Read the model definition and answer for the solid it produces. Units are mm, in the model's axes. A direction names the side the tool comes from. Give positions to 0.01 mm unless a question says otherwise; leave off trailing zeros. Order: outer loops, then holes, each group sorted by start corner. A loop starts at its lowest first (then second) coordinate and runs counter-clockwise, first axis right, second up. Notation, with made-up numbers: (62, 20) - (101, 20) arc R3 ccw to (101, 25) - close; hole circle Ø6 at (68.25, 35.5). An arc over 180 degrees is marked (long way). Answer as CSV lines item,"result". Start each with the question number.
from build123d import *

# Parameters (mm, degrees)
BOSS_EXTRUDE2_DEPTH = 5


with BuildPart() as part:
    # Sketch1 → Boss-Extrude2 (new body)
    with BuildSketch(Plane.XY):
        with BuildLine():
            Line((-28.5, 0), (-25.5, 0))
            ThreePointArc((-25.5, 0), (-24.417654986, 7.350382643), (-21.2625, 14.076792737))
            Line((-21.2625, 14.076792737), (-21.2625, 17.80655265))
            ThreePointArc((-21.2625, 17.80655265), (-20.098232577, 19.704816367), (-18.361461142, 21.098569843))
            ThreePointArc((-18.361461142, 21.098569843), (0, 25.5), (18.361461142, 21.098569843))
            ThreePointArc((18.361461142, 21.098569843), (20.098232577, 19.704816367), (21.2625, 17.80655265))
            Line((21.2625, 17.80655265), (21.2625, 14.076792737))
            ThreePointArc((21.2625, 14.076792737), (24.417654986, 7.350382643), (25.5, 0))
            Line((25.5, 0), (28.5, 0))
            ThreePointArc((28.5, 0), (27.420168216, 7.770738382), (24.2625, 14.952628322))
            Line((24.2625, 14.952628322), (24.2625, 21.105139437))
            ThreePointArc((24.2625, 21.105139437), (0, 28.5), (-24.2625, 21.105139437))
            Line((-24.2625, 21.105139437), (-24.2625, 14.952628322))
            ThreePointArc((-24.2625, 14.952628322), (-27.420168216, 7.770738382), (-28.5, 0))
        make_face()
    extrude(amount=BOSS_EXTRUDE2_DEPTH)


solid = part.part
(1) Section D-D, the plane x = 8.5 is taken. Write down the section's boundary in (y, z).
(2) Section A-A, the plane z = 3.8 is taken. Write down the section's boundary in (x, y).
(3) Section C-C, the plane y = 10 is taken. Write down the section's boundary in (x, z).
(4) Flat-ended cylindrical pins translate along their axes: pin 1 Ø1.9 at (y, z) = (15.5, 3) entering from +X; pin 2 Ø1.5 at (y, z) = (19.5, 3.5) entering from -X; pin 3 Ø2.5 at (y, z) = (17.5, 3.5) entering from +X. Find the tip coordinate at first contact, or state that the pin passes through.
(5) Straight lines are drawn through the part: line 1 (X direction, y = 16.5, z = 3.2); line 2 (X direction, y = 1.5, z = 2.45); line 3 (Y direction, x = -3.5, z = 3.2). For each, find the intervals that lie inside material, in ascending order. Write a range as [from, to].
(6) Which of the six approach directions +Z, -Z, +X, -X, +Y, -Y give full straight-line access (tool end or side, diameter ignored) to faces 4 (the cylindrical face through (27.45, 7.66, 2.46)), 5 (the flat face through (-24.262, 18, 2)), 6 (the cylindrical face through (-20.1, 19.7, 2.5))?
(7) Section B-B, the plane y = 21.75 is taken. Write down the section's boundary in (x, z).
(8) Determine the mould class of faces 1 (the flat face through (0, 26, 5)), 2 (the cylindrical face through (-0.3, 25.5, 2.5)), 3 (the flat face through (24.262, 18, 2)) for opening direction X: released by +X, released by -X, zero draft, split by the parting line, or undercut.
Checks:
1,outline,"(24.6, 0) - (27.66, 0) - (27.66, 5) - (24.6, 5) - close"
2,outline,"(-28.5, 0) - (-25.5, 0) arc R25.5 cw to (-21.26, 14.08) - (-21.26, 17.81) arc R6.5 cw to (-18.36, 21.1) arc R40.5 cw to (18.36, 21.1) arc R6.5 cw to (21.26, 17.81) - (21.26, 14.08) arc R25.5 cw to (25.5, 0) - (28.5, 0) arc R28.5 ccw to (24.26, 14.95) - (24.26, 21.11) arc R43.5 ccw to (-24.26, 21.11) - (-24.26, 14.95) arc R28.5 ccw to start"
3,outline,"(-26.69, 0) - (-23.46, 0) - (-23.46, 5) - (-26.69, 5) - close; (23.46, 0) - (26.69, 0) - (26.69, 5) - (23.46, 5) - close"
4,pin 1,"stops at x = 24.51"
4,pin 2,"stops at x = -24.26"
4,pin 3,"stops at x = 24.26"
5,line 1,"x = [-24.26, -21.26], [21.26, 24.26]"
5,line 2,"x = [-28.46, -25.46], [25.46, 28.46]"
5,line 3,"y = [25.35, 28.36]"
6,face 4,"+Z, -Z, +X, +Y"
6,face 5,"+Z, -Z, -X, +Y"
6,face 6,"+Z, -Z, -Y"
7,outline,"(-23.27, 0) - (-17.02, 0) - (-17.02, 5) - (-23.27, 5) - close; (17.02, 0) - (23.27, 0) - (23.27, 5) - (17.02, 5) - close"
8,face 1,"zero draft"
8,face 2,"undercut"
8,face 3,"released by +X"
